Autodesk Inventor part; units mm, degrees
ref_plane "YZ Plane" through (0, 0, 0) normal (1, 0, 0) x (0, 1, 0)
ref_plane "XZ Plane" through (0, 0, 0) normal (0, 1, 0) x (-1, 0, 0)
ref_plane "XY Plane" through (0, 0, 0) normal (0, 0, 1) x (1, 0, 0)
sketch "Sketch1" plane through (0, 0, 0) normal (0, 0, 1) x (1, 0, 0)
  line L0 (0, 7) -> (0, -18)
  line L1 (0, 0) -> (8, 0) construction
  arc A0 (8, 0.1689) -> (0, 7) centre (0, -1.1) ccw
  line L2 (8, 0) -> (5, 0)
  line L3 (5, 0) -> (5, -18)
  line L4 (5, -18) -> (0, -18)
  line L5 (8, 0) -> (8, 0.1689)
  dimension "d1" = 7
  dimension "d2" = 8.1
  dimension "d3" = 10
  dimension "d4" = 18
  dimension "d25" = 16
revolve "Вращение1" add sketch "Sketch1" angle 360 about axis through (0, 7, 0) along (0, -1, 0)
sketch "Sketch2" plane through (0, 0, 0) normal (0, 0, 1) x (1, 0, 0)
  line L0 (-1.25, 7) -> (1.25, 7)
  line L1 (1.25, 7) -> (1.25, 2.4)
  line L2 (1.25, 2.4) -> (-1.25, 2.4)
  line L3 (-1.25, 2.4) -> (-1.25, 7)
  line L4 (0, 0) -> (0, 7)
  arc A0 (8, 0.1689) -> (-8, 0.1689) centre (0, -1.1) ccw construction
  dimension "d6" = 2.4
  dimension "d7" = 2.5
extrude "Выдавливание1" cut sketch "Sketch2" along normal through all both and the other way through all
thread "Резьба1"
fillet "Сопряжение1" radius 0.6667 1 edges at (-5, 0, 0)
chamfer "Фаска1" distance 0.6667 angle 45 1 edges at (-5, -18, 0)
equation "\"d6\" = w"
equation "\"d7\" = n"
equation "\"d10\" = b"
equation "\"d12\" = c_"
equation "\"d13\" = c_"
equation "\"d1\" = k"
equation "\"d2\" = R1"
equation "\"d3\" = d_"
equation "\"d4\" = l_"
equation "\"d25\" = D"
equation "\"d_\" = 10"
equation "\"D\" = 16"
equation "\"k\" = 7"
equation "\"l_\" = 18"
equation "\"b\" = 18"
equation "\"n\" = 2.5"
equation "\"w\" = 2.4"
equation "\"c_\" = 0.0666667 * d_"
equation "\"R1\" = 8.1"
equation "\"G\" = 0"
properties part number "Винт A.M10-6gx18 ГОСТ 17473-80" material "Сталь, мягкая"
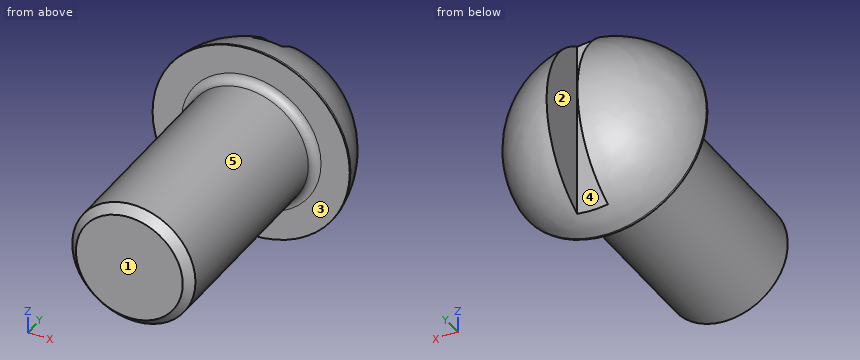
Check sheet for the modelled part. Datum: model origin and axes. Units: mm. Face numbers are marked on the shaded views. A direction names the side the tool comes from. Give positions to 0.01 mm unless a question says otherwise; leave off trailing zeros. Order: outer loops, then holes, each group sorted by start corner. A loop starts at its lowest first (then second) coordinate and runs counter-clockwise, first axis right, second up. Notation, with made-up numbers: (41.25, 10.5) -> (70.25, 10.5) arc R33 ccw to (70.25, 38.5) -> close; hole circle Ø11 at (83.5, -7). An arc over 180 degrees is marked (long way). Return JSON: item names as keys, results as strings.
1. Material ranges on probe 1 along Z at (x, y) = (-0.25, -10.25); probe 2 along Y at (x, z) = (0.5, 3); probe 3 along X at (y, z) = (3.5, 3.5), recorded low to high. Write a range as [from, to].
From the geometry:
{"probe 1": "[-4.99, 4.99]", "probe 2": "[-18, 2.4]", "probe 3": "[-5.67, -1.25], [1.25, 5.67]"}
2. Go/stop test with flat-tipped pins: P1, Ø1.3, axis at x = 0.5, z = 3, coming from the +Y side; P2, Ø8, axis at x = 0, z = -5.5, coming from the +Y side; P3, Ø6, axis at y = -15.5, z = -2, coming from the +X side. Record where each tip stops, or that it passes through.
From the geometry:
{"P1": "y = 2.4", "P2": "y = 6.72", "P3": "x = 5"}
3. Mould release check, pull along X, two halves, no side actions. Record for the marked faces 3, 4 and 5: +X half, -X half, draft (parallel to the pull), parting line (faces both ways), or undercut.
From the geometry:
{"face 3": "draft", "face 4": "undercut", "face 5": "parting line"}
4. Set-up check for the marked faces 1 and 2: record each of +Z, -Z, +X, -X, +Y, -Y from which the full face is reachable in a straight line by a thin tool's end or side.
From the geometry:
{"face 1": "+Z, -Z, +X, -X, -Y", "face 2": "+Z, -Z, +Y"}
5. Cross-section at A-A, the plane y = -15.75. Record the cut outline in (x, z), plus the area to 3 significant figures.
From the geometry:
{"outline": "circle Ø10 at (0, 0)", "area": "78.5 mm^2"}
